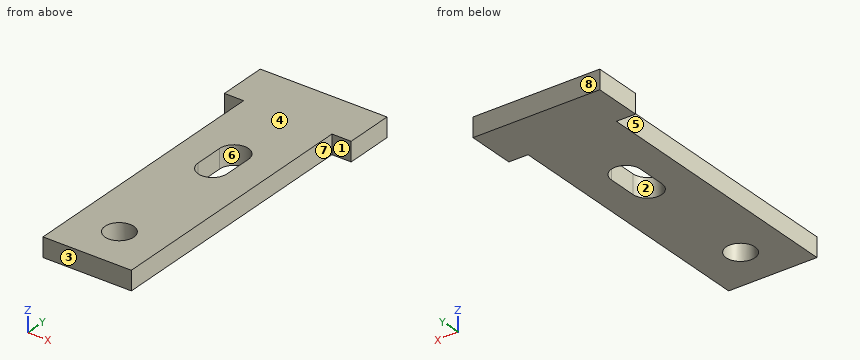
```python
from build123d import *

# Parameters (mm, degrees)
SKETCH1_W           = 11.684
SKETCH1_H           = 2.54
BOSS_EXTRUDE1_DEPTH = 35.56
BOSS_EXTRUDE2_DEPTH = 2.54
CUT_EXTRUDE1_REACH  = 4.54
SKETCH3_R           = 1.905


with BuildPart() as part:
    # Sketch1 → Boss-Extrude1 (new body)
    with BuildSketch(Plane(origin=(0, 0, 0), x_dir=(1, 0, 0), z_dir=(0, 1, 0))):
        Rectangle(SKETCH1_W, SKETCH1_H)
    extrude(amount=BOSS_EXTRUDE1_DEPTH)

    # Sketch2 → Boss-Extrude2 (add)
    with BuildSketch(Plane.XY.offset(1.27)):
        Polygon((-8.382, 35.56), (-5.842, 35.56), (5.842, 35.56), (8.382, 35.56), (8.382, 41.91), (-8.382, 41.91), align=None)
    extrude(amount=-BOSS_EXTRUDE2_DEPTH)

    # Sketch3 → Cut-Extrude1 (cut, up to next)
    with BuildSketch(Plane.XY.offset(1.27), mode=Mode.PRIVATE) as cut_extrude1_sk1:
        with Locations((0, 5.715)):
            Circle(SKETCH3_R)
    cut_extrude1_tool1 = extrude(cut_extrude1_sk1.sketch, amount=-CUT_EXTRUDE1_REACH, mode=Mode.PRIVATE) & part.part
    add(cut_extrude1_tool1.solids().sort_by_distance((0, 5.715, 1.27))[0], mode=Mode.SUBTRACT)
    # Sketch3 → Cut-Extrude1 (cut, up to next)
    with BuildSketch(Plane.XY.offset(1.27), mode=Mode.PRIVATE) as cut_extrude1_sk2:
        with BuildLine():
            Line((1.905, 26.035), (1.905, 22.225))
            ThreePointArc((1.905, 22.225), (0, 20.32), (-1.905, 22.225))
            Line((-1.905, 22.225), (-1.905, 26.035))
            ThreePointArc((-1.905, 26.035), (0, 27.94), (1.905, 26.035))
        make_face()
    cut_extrude1_tool2 = extrude(cut_extrude1_sk2.sketch, amount=-CUT_EXTRUDE1_REACH, mode=Mode.PRIVATE) & part.part
    add(cut_extrude1_tool2.solids().sort_by_distance((0, 24.13, 1.27))[0], mode=Mode.SUBTRACT)


solid = part.part
```
Build history of the part. All positions in model axes, mm. Face numbers are marked on the shaded views. A direction names the side the tool comes from. Coordinates: 2 decimals unless noted, no trailing zeros. Order: outer loops, then holes, each group sorted by start corner. A loop starts at its lowest first (then second) coordinate and runs counter-clockwise, first axis right, second up. Notation, with made-up numbers: M -28,14.5 L 31,14.5 A33 ccw 31,47.5 Z; hole C 12,-18 d5. An arc over 180 degrees is marked long. One line per question, with ' | ' between items. Start each with the question number.
1. Mould opens along X. For the marked faces 6, 7 and 8 say: +X half, -X half, draft (parallel to the pull), parting line (faces both ways), or undercut.
2. Cut at D-D (y = 30.5). Write the cut outline in (x, z), plus the area to 3 significant figures.
3. Tool access for the marked faces 1, 2, 3, 4 and 5: list every direction of +Z, -Z, +X, -X, +Y, -Y with a clear straight run to the whole face (end or side of a thin tool).
4. Cut at A-A (x = 0). Write the cut outline in (y, z).
5. Cut at B-B (y = 23.5). Write the cut outline in (x, z) (3 decimals), plus the area to 3 significant figures.
6. Wall check: line 1 along Y through (x, z) = (0, -0.05); line 2 along Y through (x, z) = (-6.5, 0.35); line 3 along X through (y, z) = (30.5, 0.9). Give the ranges that are in metal, low to high. Write a range as [from, to].
7. Flat gauge pins, fed straight in: P1, Ø5, axis at x = 6.5, y = 33, coming from the +Z side; P2, Ø1.3, axis at x = -7.5, z = -0.5, coming from the -Y side; P3, Ø1.3, axis at y = 24.5, z = 0, coming from the +X side; P4, Ø1.5, axis at y = 16, z = -1, coming from the -X side. Where does each tip first touch, or does it go through?
8. Cut at C-C (z = -0.1). Write the cut outline in (x, y) (3 decimals), plus the area to 3 significant figures.
The answers:
1) face 6: undercut | face 7: +X half | face 8: draft
2) outline: M -5.84,-1.27 L 5.84,-1.27 L 5.84,1.27 L -5.84,1.27 Z | area: 29.7 mm2
3) face 1: +Z, -Z, +X, -Y | face 2: +Z, -Z | face 3: +Z, -Z, +X, -X, -Y | face 4: +Z, +X, -X, +Y, -Y | face 5: +Z, -Z, -X, -Y
4) outline: M 0,-1.27 L 3.81,-1.27 L 3.81,1.27 L 0,1.27 Z; M 7.62,-1.27 L 20.32,-1.27 L 20.32,1.27 L 7.62,1.27 Z; M 27.94,-1.27 L 41.91,-1.27 L 41.91,1.27 L 27.94,1.27 Z
5) outline: M -5.842,-1.27 L -1.905,-1.27 L -1.905,1.27 L -5.842,1.27 Z; M 1.905,-1.27 L 5.842,-1.27 L 5.842,1.27 L 1.905,1.27 Z | area: 20.0 mm2
6) line 1: y = [0, 3.81], [7.62, 20.32], [27.94, 41.91] | line 2: y = [35.56, 41.91] | line 3: x = [-5.84, 5.84]
7) P1: stops at z = 1.27 | P2: stops at y = 35.56 | P3: stops at x = 5.84 | P4: stops at x = -5.84
8) outline: M -8.382,35.56 L -5.842,35.56 L -5.842,0 L 5.842,0 L 5.842,35.56 L 8.382,35.56 L 8.382,41.91 L -8.382,41.91 Z; hole C 0,5.715 d3.81; hole M -1.905,22.225 A1.905 ccw 1.905,22.225 L 1.905,26.035 A1.905 ccw -1.905,26.035 Z | area: 485 mm2
